The drawing under review shows one solid part. Ordinate dimensions are in mm from its lowest x, y, z. A direction names the side the tool comes from. Give positions to 0.01 mm unless a question says otherwise; leave off trailing zeros. Write each loop counter-clockwise with the first axis right and the second up, starting at its lowest first coordinate (ties: lowest second). Pieces come first, ordered by that corner, then holes. Notation, with made-up numbers: (19, -25.75) - (50, -25.75) arc R31 cw to (50, 8.25) - close; hole circle Ø7 at (-17, 6). An arc over 180 degrees is marked (long way). Write item = value, one per line.
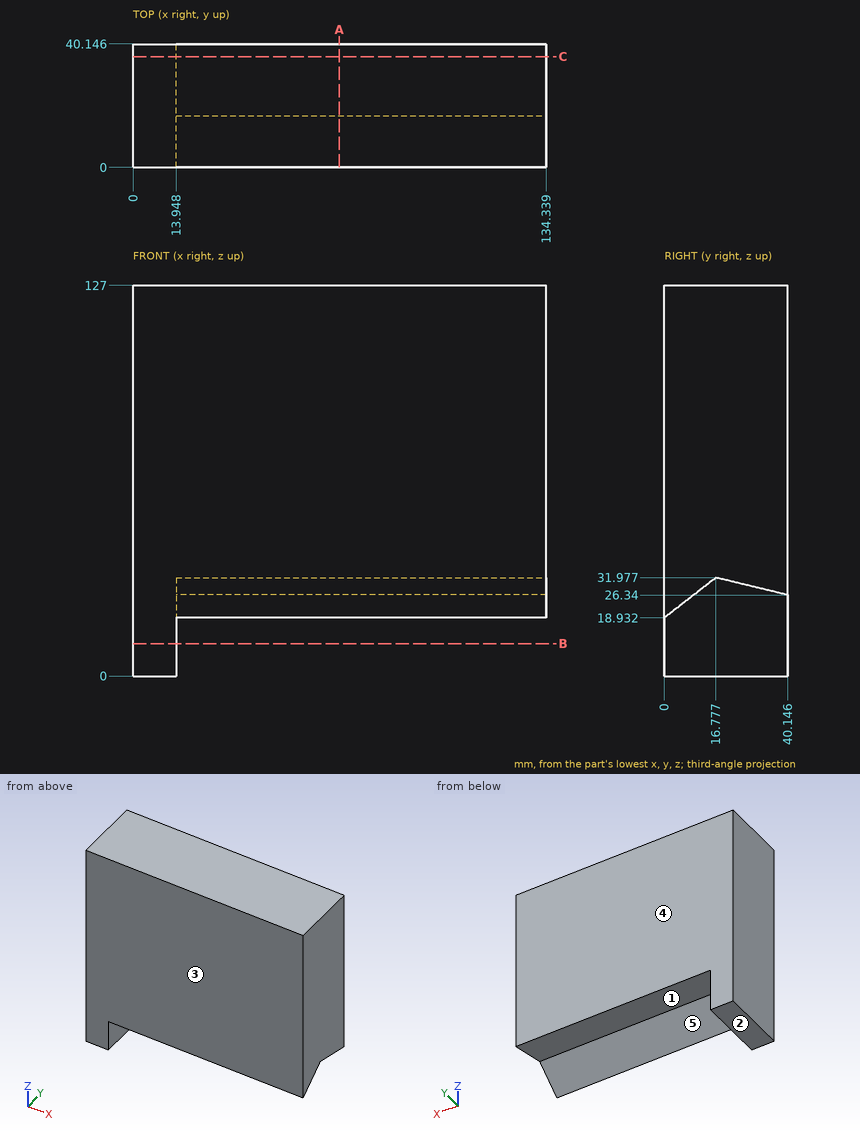
1. Machinability: for the marked faces 4 and 5, which of the approach directions +Z, -Z, +X, -X, +Y, -Y give a long, thin tool a straight path to every point of the face, cutting with its end or side? Answer none if there is none.
Findings below:
face_4 = +Z, -Z, +X, -X, +Y
face_5 = -Z, +X
2. For line 1 (X direction, y = 35.5, z = 19.5); line 2 (Z direction, x = 61, y = 3) (1 decimal); line 3 (Z direction, x = 57, y = 34.5), list the stretches that pass through material, from the lowest coordinate up. Write a range as from..to.
Findings below:
line_1 = 0..13.95
line_2 = 21.3..127
line_3 = 27.7..127
3. Take a section at A-A on x = 67. Give the boundary of the cut face in (y, z) (1 decimal).
Findings below:
outline = (0, 18.9) - (16.8, 32) - (40.1, 26.3) - (40.1, 127) - (0, 127) - close
4. Take a section at B-B on z = 10.5. Give the boundary of the cut face in (x, y) (1 decimal).
Findings below:
outline = (0, 0) - (13.9, 0) - (13.9, 40.1) - (0, 40.1) - close
5. Draft analysis for pull direction Y (two halves, no side actions). For the marked faces 1, 2 and 3, state which applies: +Y half, -Y half, draft (parallel to the pull), parting line (faces both ways), or undercut.
Findings below:
face_1 = undercut
face_2 = draft
face_3 = -Y half
6. Insertion check: P1, Ø1.5, axis at x = 61.5, y = 23, coming from the -Z side (1 decimal); P2, Ø1, axis at x = 20.5, y = 8, coming from the -Z side (1 decimal); P3, Ø9.5, axis at y = 18.5, z = 21.5, coming from the +X side. Each pin has a flat end and moves straight along its axis. Give the tip position at first contact, or say it passes through.
Findings below:
P1 = 30.3
P2 = 24.8
P3 = 13.95
7. Take a section at C-C on y = 36. Give the boundary of the cut face in (x, z), and give its area (3 significant figures).
Findings below:
outline = (0, 0) - (13.95, 0) - (13.95, 27.34) - (134.34, 27.34) - (134.34, 127) - (0, 127) - close
area = 13,800 mm²
